Geometry check sheet. Reference: the model listing, model coordinates, mm. Face numbers are marked on the shaded views. Coordinates: 2 decimals unless noted, no trailing zeros. Write each loop counter-clockwise with the first axis right and the second up, starting at its lowest first coordinate (ties: lowest second). Pieces come first, ordered by that corner, then holes. Notation, with made-up numbers: (78, 60.25) -> (101, 60.25) arc R17 ccw to (101, 69.25) -> close; hole circle Ø6 at (65.25, -23.5). An arc over 180 degrees is marked (long way). Answer in a Markdown table with one row per item. Add a question column.
1. Cross-section at A-A on x = -40.5. Record the cut outline in (y, z) (1 decimal).
2. Mould release check, pull along Y, two halves, no side actions. Record for the marked faces 1 and 2: pulls with the +Y half, pulls with the -Y half, needs draft (parallel to the pull), parting line crosses it, or undercut.
3. Cross-section at B-B on z = 92. Record the cut outline in (x, y) (3 decimals), and give its area (3 significant figures).
4. Depth check by flat-ended pin: P1, Ø1, axis at y = 1, z = 44.5, coming from the +X side (3 decimals); P2, Ø1, axis at y = 1, z = -64, coming from the -X side (3 decimals); P3, Ø10, axis at x = -21.5, z = 19, coming from the +Y side (3 decimals). Enter the tip coordinate at first touch or a pass-through.
5. Cross-section at C-C on z = -21.59. Record the cut outline in (x, y) (3 decimals).
6. Scan lines: L1, parallel to Z at x = -17, y = 1.8; L2, parallel to X at y = 2.4, z = 55 (3 decimals); L3, parallel to Z at x = 67, y = 2.1. Record each from-to range of solid material in increasing order. Write a range as from..to.
7. Cross-section at D-D on y = 1.55. Give the number of separate pieces and of enclosed holes in the cut face, and give its area (3 significant figures).
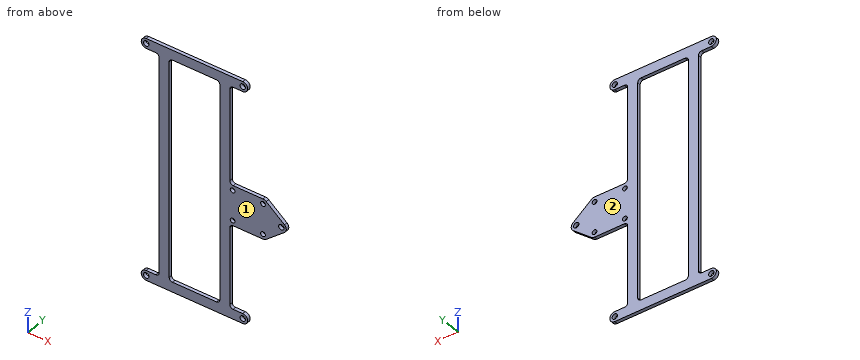
Autodesk Inventor part; units mm, degrees
ref_plane "YZ Plane" through (0, 0, 0) normal (1, 0, 0) x (0, 1, 0)
ref_plane "XZ Plane" through (0, 0, 0) normal (0, 1, 0) x (-1, 0, 0)
ref_plane "XY Plane" through (0, 0, 0) normal (0, 0, 1) x (1, 0, 0)
sketch "Sketch1" plane through (0, 0, 0) normal (0, 1, 0) x (-1, 0, 0)
  line L0 (45.974, 111.125) -> (-45.974, 111.125) construction
  line L1 (45.974, 115.8875) -> (-45.974, 115.8875)
  line L2 (-45.974, 106.3625) -> (45.974, 106.3625)
  arc A0 (45.974, 106.3625) -> (45.974, 115.8875) centre (45.974, 111.125) ccw
  arc A1 (-45.974, 115.8875) -> (-45.974, 106.3625) centre (-45.974, 111.125) ccw
  line L3 (0, 111.125) -> (0, -111.125) construction
  line L4 (45.974, -111.125) -> (-45.974, -111.125) construction
  line L5 (45.974, -115.8875) -> (-45.974, -115.8875)
  line L6 (-45.974, -106.3625) -> (45.974, -106.3625) construction
  arc A2 (45.974, -115.8875) -> (45.974, -106.3625) centre (45.974, -111.125) ccw
  arc A3 (-45.974, -106.3625) -> (-45.974, -115.8875) centre (-45.974, -111.125) ccw
  line L7 (24.13, 106.3625) -> (24.13, -106.3625)
  line L8 (-24.13, 106.3625) -> (-24.13, -106.3625) construction
  line L9 (24.13, 0) -> (-24.13, 0) construction
  line L10 (33.655, 106.3625) -> (33.655, -106.3625)
  line L11 (-33.655, 106.3625) -> (-33.655, -106.3625)
  line L12 (45.974, -106.3625) -> (33.655, -106.3625)
  line L13 (-24.13, -106.3625) -> (24.13, -106.3625)
  line L14 (-24.13, -106.3625) -> (-24.13, 106.3625)
  line L15 (-33.655, -106.3625) -> (-45.974, -106.3625)
  line L16 (14.478, 14.478) -> (-14.478, -14.478) construction
  circle A4 centre (14.478, 14.478) radius 4.7625 construction
  circle A5 centre (-14.478, -14.478) radius 4.7625 construction
  line L17 (11.1788, 17.9127) -> (24.13, 30.353)
  line L18 (11.1788, 11.0433) -> (24.13, -1.397)
  line L19 (-11.1788, -17.9127) -> (-24.13, -30.353)
  line L20 (-11.1788, -11.0433) -> (-24.13, 1.397)
  arc A6 (11.1788, 17.9127) -> (11.1788, 11.0433) centre (14.478, 14.478) ccw
  arc A7 (-11.1788, -17.9127) -> (-11.1788, -11.0433) centre (-14.478, -14.478) ccw
  point P0 (0, 0)
  point P1 (0, 0)
  point P2 (0, 0)
  point P3 (-33.655, 106.3625)
  point P4 (33.655, 106.3625)
  point P5 (0, 0)
  dimension "d0" = 9.525
  dimension "d1" = 91.948
  dimension "d2" = 222.25
  dimension "d4" = 9.525
  dimension "d5" = 48.26
  dimension "d6" = 9.525
  dimension "d7" = 9.525
  dimension "d33" = 28.956
  dimension "d34" = 28.956
  dimension "d35" = 9.525
  dimension "d36" = 9.525
  dimension "d37" = 15.875
  dimension "d38" = 15.875
  dimension "d39" = 15.875
  dimension "d40" = 15.875
extrude "Extrusion1" add sketch "Sketch1" along normal blind 3.175 contours A0 L2 A1 L1 | L10 L12 A2 L5 A3 L15 L11 L2 L14 L13 L7
sketch "Sketch2" plane through (0, 3.175, 0) normal (0, 1, 0) x (1, 0, 0)
  line L0 (-33.655, -106.3625) -> (-45.974, -106.3625) construction
  arc A0 (-45.974, -106.3625) -> (-45.974, -115.8875) centre (-45.974, -111.125) ccw construction
  line L1 (-45.974, -115.8875) -> (45.974, -115.8875) construction
  arc A1 (45.974, -115.8875) -> (45.974, -106.3625) centre (45.974, -111.125) ccw construction
  line L2 (-24.13, -106.3625) -> (-24.13, 106.3625)
  line L3 (-24.13, 106.3625) -> (24.13, 106.3625)
  line L4 (24.13, 106.3625) -> (24.13, -106.3625)
  line L5 (24.13, -106.3625) -> (-24.13, -106.3625)
  line L6 (45.974, -106.3625) -> (33.655, -106.3625)
  line L7 (33.655, -106.3625) -> (33.655, 106.3625)
  line L8 (33.655, 106.3625) -> (45.974, 106.3625)
  arc A2 (45.974, 106.3625) -> (45.974, 115.8875) centre (45.974, 111.125) ccw
  line L9 (45.974, 115.8875) -> (-45.974, 115.8875)
  arc A3 (-45.974, 115.8875) -> (-45.974, 106.3625) centre (-45.974, 111.125) ccw
  line L10 (-45.974, 106.3625) -> (-33.655, 106.3625)
  line L11 (-33.655, 106.3625) -> (-33.655, -106.3625)
  point P0 (0, 0)
  point P1 (45.974, 111.125)
  point P2 (-45.974, 111.125)
  point P3 (-14.478, 71.0565)
  point P4 (14.478, 100.0125)
hole "Hole1" at (-45.974, 3.175, 111.125) at (45.974, 3.175, 111.125) at (45.974, 3.175, -111.125) at (-45.974, 3.175, -111.125) direction (0, -1, 0) diameter 5.1054 end through all
sketch "Sketch3" plane through (0, 3.175, 0) normal (0, 1, 0) x (1, 0, 0)
  circle A0 centre (45.974, 111.125) radius 2.5527 construction
  circle A1 centre (-45.974, -111.125) radius 2.5527 construction
  circle A2 centre (45.974, -111.125) radius 2.5527 construction
  circle A3 centre (-45.974, 111.125) radius 2.5527 construction
  line L0 (-24.13, -106.3625) -> (24.13, -106.3625) construction
  line L1 (24.13, -106.3625) -> (24.13, 106.3625) construction
  line L2 (24.13, 106.3625) -> (-24.13, 106.3625) construction
  line L3 (-24.13, 106.3625) -> (-24.13, -106.3625) construction
  line L4 (-33.655, -106.3625) -> (-33.655, 106.3625) construction
  line L5 (-33.655, 106.3625) -> (-45.974, 106.3625) construction
  arc A4 (-45.974, 115.8875) -> (-45.974, 106.3625) centre (-45.974, 111.125) ccw construction
  line L6 (-45.974, 115.8875) -> (45.974, 115.8875) construction
  arc A5 (45.974, 106.3625) -> (45.974, 115.8875) centre (45.974, 111.125) ccw construction
  line L7 (45.974, 106.3625) -> (33.655, 106.3625) construction
  line L8 (33.655, 106.3625) -> (33.655, -106.3625) construction
  line L9 (33.655, -106.3625) -> (45.974, -106.3625) construction
  arc A6 (45.974, -115.8875) -> (45.974, -106.3625) centre (45.974, -111.125) ccw construction
  line L10 (45.974, -115.8875) -> (-45.974, -115.8875) construction
  arc A7 (-45.974, -106.3625) -> (-45.974, -115.8875) centre (-45.974, -111.125) ccw construction
  line L11 (-45.974, -106.3625) -> (-33.655, -106.3625) construction
  line L12 (65.278, -7.366) -> (36.322, 21.59) construction
  circle A8 centre (65.278, -7.366) radius 4.7625 construction
  circle A9 centre (36.322, 21.59) radius 4.7625 construction
  line L13 (33.655, -106.3625) -> (33.655, 106.3625) construction
  circle A10 centre (36.322, -7.366) radius 4.7625 construction
  circle A11 centre (65.278, 21.59) radius 4.7625 construction
  line L14 (33.655, -12.1285) -> (65.278, -12.1285)
  line L15 (70.0405, -7.366) -> (70.0405, 21.59)
  line L16 (65.278, 26.3525) -> (33.655, 26.3525)
  arc A12 (65.278, -12.1285) -> (70.0405, -7.366) centre (65.278, -7.366) ccw
  arc A13 (70.0405, 21.59) -> (65.278, 26.3525) centre (65.278, 21.59) ccw
  line L17 (33.655, -12.1285) -> (33.655, 26.3525)
  point P0 (0, 0)
  point P1 (50.8, 7.112)
  dimension "d48" = 31.623
  dimension "d50" = 28.956
  dimension "d51" = 9.525
  dimension "d66" = 7.112
  dimension "d67" = 28.956
extrude "Extrusion2" add sketch "Sketch3" against normal blind 3.175
fillet "Fillet2" radius 3.302 2 edges at (33.655, 1.5875, 12.1285) (33.655, 1.5875, -26.3525)
hole "Hole4" at (65.278, 3.175, 7.366) at (36.322, 3.175, -21.59) at (36.322, 3.175, 7.366) at (65.278, 3.175, -21.59) direction (0, -1, 0) diameter 4.4958 end through all
sketch "Sketch5" plane through (0, 3.175, 0) normal (0, 1, 0) x (1, 0, 0)
  circle A0 centre (82.7405, 7.112) radius 4.7625 construction
  circle A1 centre (36.322, -7.366) radius 2.2479 construction
  circle A2 centre (65.278, -7.366) radius 2.2479 construction
  circle A3 centre (36.322, 21.59) radius 2.2479 construction
  circle A4 centre (65.278, 21.59) radius 2.2479 construction
  circle A5 centre (45.974, 111.125) radius 2.5527 construction
  circle A6 centre (-45.974, -111.125) radius 2.5527 construction
  circle A7 centre (45.974, -111.125) radius 2.5527 construction
  circle A8 centre (-45.974, 111.125) radius 2.5527 construction
  line L0 (-24.13, -106.3625) -> (24.13, -106.3625) construction
  line L1 (24.13, -106.3625) -> (24.13, 106.3625) construction
  line L2 (24.13, 106.3625) -> (-24.13, 106.3625) construction
  line L3 (-24.13, 106.3625) -> (-24.13, -106.3625) construction
  line L4 (-33.655, -106.3625) -> (-33.655, 106.3625) construction
  line L5 (-33.655, 106.3625) -> (-45.974, 106.3625) construction
  arc A9 (-45.974, 115.8875) -> (-45.974, 106.3625) centre (-45.974, 111.125) ccw construction
  line L6 (-45.974, 115.8875) -> (45.974, 115.8875) construction
  arc A10 (45.974, 106.3625) -> (45.974, 115.8875) centre (45.974, 111.125) ccw construction
  line L7 (45.974, 106.3625) -> (33.655, 106.3625) construction
  line L8 (33.655, 106.3625) -> (33.655, 29.6545) construction
  arc A11 (33.655, 29.6545) -> (36.957, 26.3525) centre (36.957, 29.6545) ccw construction
  line L9 (36.957, 26.3525) -> (65.278, 26.3525) construction
  arc A12 (70.0405, 21.59) -> (65.278, 26.3525) centre (65.278, 21.59) ccw construction
  line L10 (70.0405, 21.59) -> (70.0405, -7.366) construction
  arc A13 (65.278, -12.1285) -> (70.0405, -7.366) centre (65.278, -7.366) ccw construction
  line L11 (65.278, -12.1285) -> (36.957, -12.1285) construction
  arc A14 (36.957, -12.1285) -> (33.655, -15.4305) centre (36.957, -15.4305) ccw construction
  line L12 (33.655, -15.4305) -> (33.655, -106.3625) construction
  line L13 (33.655, -106.3625) -> (45.974, -106.3625) construction
  arc A15 (45.974, -115.8875) -> (45.974, -106.3625) centre (45.974, -111.125) ccw construction
  line L14 (45.974, -115.8875) -> (-45.974, -115.8875) construction
  arc A16 (-45.974, -106.3625) -> (-45.974, -115.8875) centre (-45.974, -111.125) ccw construction
  line L15 (-45.974, -106.3625) -> (-33.655, -106.3625) construction
  arc A17 (70.0405, 21.59) -> (65.278, 26.3525) centre (65.278, 21.59) ccw construction
  line L16 (68.3177, 25.2563) -> (85.7802, 10.7783)
  line L17 (85.7802, 3.4457) -> (68.3177, -11.0323)
  arc A18 (85.7802, 3.4457) -> (85.7802, 10.7783) centre (82.7405, 7.112) ccw
  line L18 (70.0405, 21.59) -> (70.0405, -7.366)
  arc A19 (70.0405, 21.59) -> (68.3177, 25.2563) centre (65.278, 21.59) ccw
  arc A20 (65.278, -12.1285) -> (70.0405, -7.366) centre (65.278, -7.366) ccw construction
  arc A21 (68.3177, -11.0323) -> (70.0405, -7.366) centre (65.278, -7.366) ccw
  point P0 (0, 0)
  point P1 (70.0405, 7.112)
  point P2 (70.0405, -7.366)
  dimension "d76" = 9.525
  dimension "d77" = 12.7
extrude "Extrusion3" add sketch "Sketch5" against normal up to surface (3.175 mm away)
hole "Hole6" at (82.7405, 3.175, -7.112) direction (0, -1, 0) diameter 5.1054 end through all
fillet "Fillet3" radius 3.175 8 edges at (-24.13, 1.5875, -106.3625) (24.13, 1.5875, -106.3625) (-33.655, 1.5875, -106.3625) (33.655, 1.5875, -106.3625) (-33.655, 1.5875, 106.3625) (-24.13, 1.5875, 106.3625) (24.13, 1.5875, 106.3625) (33.655, 1.5875, 106.3625)
equation "\"d4\" = d0"
equation "\"d6\" = d7"
equation "\"d38\" = d37"
equation "\"d39\" = d37"
equation "\"d40\" = d39"
properties part number "DB1-007" material "Aluminum 6061"
Results found:
| question | item | result |
|---|---|---|
| 1 | outline | (0, -115.9) -> (3.2, -115.9) -> (3.2, -106.4) -> (0, -106.4) -> close; (0, 106.4) -> (3.2, 106.4) -> (3.2, 115.9) -> (0, 115.9) -> close |
| 2 | face 1 | pulls with the -Y half |
| 2 | face 2 | pulls with the +Y half |
| 3 | outline | (-33.655, 0) -> (-24.13, 0) -> (-24.13, 3.175) -> (-33.655, 3.175) -> close; (24.13, 0) -> (33.655, 0) -> (33.655, 3.175) -> (24.13, 3.175) -> close |
| 3 | area | 60.5 mm^2 |
| 4 | P1 | stops at x = 33.655 |
| 4 | P2 | stops at x = -33.655 |
| 4 | P3 | stops at y = 3.175 |
| 5 | outline | (-33.655, 0) -> (-24.13, 0) -> (-24.13, 3.175) -> (-33.655, 3.175) -> close; (24.13, 0) -> (34.074, 0) -> (34.074, 3.175) -> (24.13, 3.175) -> close; (38.57, 0) -> (63.03, 0) -> (63.03, 3.175) -> (38.57, 3.175) -> close; (67.526, 0) -> (72.74, 0) -> (72.74, 3.175) -> (67.526, 3.175) -> close |
| 6 | L1 | z = -115.89..-106.36, 106.36..115.89 |
| 6 | L2 | x = -33.655..-24.13, 24.13..33.655 |
| 6 | L3 | z = -26.03..-23.03, -20.15..5.92, 8.81..11.81 |
| 7 | separate pieces | 1 |
| 7 | enclosed holes | 10 |
| 7 | area | 7,520 mm^2 |
